from build123d import *

# Parameters (mm, degrees)
F0_R     = 5.5
F0_W     = 48
F0_H     = 82
F1_DEPTH = 16
F3_DEPTH = 82.001


with BuildPart() as f1:
    # F0 (on Top) → F1 (new body)
    with BuildSketch(Plane.XY):
        with BuildLine():
            Line((0, 68), (0, 14))
            ThreePointArc((0, 14), (4.100505, 4.100505), (14, 0))
            Line((14, 0), (44, 0))
            Line((44, 0), (44, 82))
            Line((44, 82), (14, 82))
            ThreePointArc((14, 82), (4.100505, 77.899495), (0, 68))
        make_face()
        with Locations((14, 14)):
            Circle(F0_R, mode=Mode.SUBTRACT)
        with Locations((14, 68)):
            Circle(F0_R, mode=Mode.SUBTRACT)
        with Locations((68, 41)):
            Rectangle(F0_W, F0_H)
        with BuildLine():
            Line((92, 82), (92, 0))
            Line((92, 0), (122, 0))
            ThreePointArc((122, 0), (131.899495, 4.100505), (136, 14))
            Line((136, 14), (136, 68))
            ThreePointArc((136, 68), (131.899495, 77.899495), (122, 82))
            Line((122, 82), (92, 82))
        make_face()
        with Locations((121.999683, 14.261592)):
            Circle(F0_R, mode=Mode.SUBTRACT)
        with Locations((121.999683, 68.261592)):
            Circle(F0_R, mode=Mode.SUBTRACT)
    extrude(amount=F1_DEPTH)

    # F2 (on Front) → F3 (intersect, through all)
    with BuildSketch(Plane.XZ):
        with BuildLine():
            Line((0, 16), (0, 4))
            Line((0, 4), (38, 4))
            Line((38, 4), (38, 0))
            Line((38, 0), (98, 0))
            Line((98, 0), (98, 4))
            Line((98, 4), (136, 4))
            Line((136, 4), (136, 16))
            Line((136, 16), (92, 16))
            ThreePointArc((92, 16), (91.110896, 13.447605), (88.828427, 12))
            Line((88.828427, 12), (46.828427, 12))
            ThreePointArc((46.828427, 12), (44.378937, 13.267949), (44, 16))
            Line((44, 16), (0, 16))
        make_face()
    extrude(amount=-F3_DEPTH, mode=Mode.INTERSECT)


solid = f1.part
Can you work these out from the model? Positions are in its coordinate system, mm. A direction names the side the tool comes from. Round coordinates to 2 decimals unless told otherwise and drop trailing zeros. Loops run counter-clockwise (first coordinate to the right, second up) from the corner with the lowest first, then second, coordinate; pieces in that order, holes last. Notation, with made-up numbers: (21, -13.5) - (59, -13.5) arc R31 ccw to (59, 11.5) - close; hole circle Ø8 at (-20, 0). An arc over 180 degrees is marked (long way). Write item = value, one per line. Start each with the question number.
(1) For faces 1 (the face through (38, 40, 2)), 2 (the face through (98, 40, 2)), 3 (the face through (68, 40, 12)), which set-ups out of +Z, -Z, +X, -X, +Y, -Y let a thin tool reach every point of the face, with its end or its side?
(2) For P1, Ø1.2, axis at y = 30, z = 1.5, coming from the -X side; P2, Ø19, axis at x = 27.5, y = 27.5, coming from the -Z side; P3, Ø21, axis at x = 58, y = 26.5, coming from the +Z side; P4, Ø9, axis at x = 14, y = 68, coming from the +Z side, each with a flat end and sliding along its axis, tell me the tip position at first contact or that it passes through.
(3) If we section it at A-A (y = 61): Please give me the cut outline in (x, z).
(4) If we mould it in two halves opening along Y, with no side actions, what happens to faces 4 (the face through (91.135, 40.426, 13.478)), 5 (the face through (4.2, 78, 9.9)), 6 (the face through (131.8, 4, 9.9)), 7 (the face through (116.505, 68.503, 9.916))? For each: released by +Y, released by -Y, zero draft, split by the parting line, or undercut.
(5) If I drill on probe 1 along Y at (x, z) = (14, 13.25); probe 2 along Y at (x, z) = (16, 15.5); probe 3 along Z at (x, y) = (21, 32), over which ranges is the centre line in solid material (lowest first)? Write a range as [from, to].
(6) If we section it at B-B (z = 6.5): Please give me the cut outline in (x, y).
(7) If we section it at C-C (x = 65): Please give me the cut outline in (y, z), and give its area (3 significant figures).
Ans:
q1.face_1 = -Z, -X, +Y, -Y
q1.face_2 = -Z, +X, +Y, -Y
q1.face_3 = +Z, +Y, -Y
q2.P1 = 38
q2.P2 = 4
q2.P3 = 12
q2.P4 = through
q3.outline = (0, 4) - (38, 4) - (38, 0) - (98, 0) - (98, 4) - (136, 4) - (136, 16) - (92, 16) arc R4.11 cw to (88.83, 12) - (46.83, 12) arc R3 cw to (44, 16) - (0, 16) - close
q4.face_4 = zero draft
q4.face_5 = released by +Y
q4.face_6 = released by -Y
q4.face_7 = undercut
q5.probe_1 = [0, 8.5], [19.5, 62.5], [73.5, 82]
q5.probe_2 = [0, 8.88], [19.12, 62.88], [73.12, 82]
q5.probe_3 = [4, 16]
q6.outline = (0, 14) arc R14 ccw to (14, 0) - (122, 0) arc R14 ccw to (136, 14) - (136, 68) arc R14 ccw to (122, 82) - (14, 82) arc R14 ccw to (0, 68) - close; hole circle Ø11 at (14, 14); hole circle Ø11 at (14, 68); hole circle Ø11 at (122, 14.26); hole circle Ø11 at (122, 68.26)
q7.outline = (0, 0) - (82, 0) - (82, 12) - (0, 12) - close
q7.area = 984 mm²
